Source: three-view drawing plus pictorial views. Frame: mm from the lowest corner of the part. A direction names the side the tool comes from. Coordinates: 2 decimals unless noted, no trailing zeros. Write each loop counter-clockwise with the first axis right and the second up, starting at its lowest first coordinate (ties: lowest second). Pieces come first, ordered by that corner, then holes. Notation, with made-up numbers: (19, 3.5) -> (55, 3.5) arc R22 ccw to (55, 29.5) -> close; hole circle Ø8 at (-15, 2). An arc over 180 degrees is marked (long way). One line per item, written item: value.
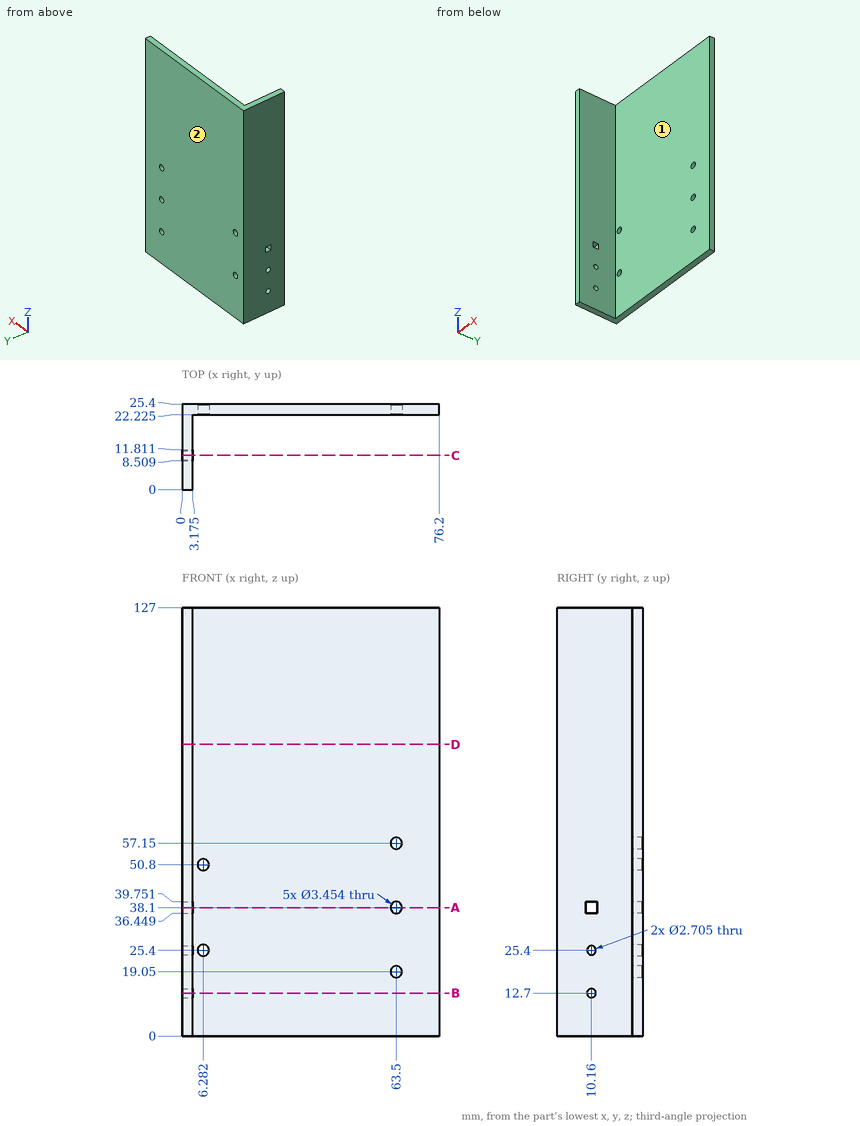
(1) Section C-C (y = 10.16). Return the cut outline in (x, z) (1 decimal).
Responses:
outline: (0, 0) -> (3.2, 0) -> (3.2, 11.3) -> (0, 11.3) -> close; (0, 14.1) -> (3.2, 14.1) -> (3.2, 24) -> (0, 24) -> close; (0, 26.8) -> (3.2, 26.8) -> (3.2, 36.4) -> (0, 36.4) -> close; (0, 39.8) -> (3.2, 39.8) -> (3.2, 127) -> (0, 127) -> close
(2) Section B-B (z = 12.7). Return the cut outline in (x, y) (1 decimal).
Responses:
outline: (0, 0) -> (3.2, 0) -> (3.2, 8.8) -> (0, 8.8) -> close; (0, 11.5) -> (3.2, 11.5) -> (3.2, 22.2) -> (76.2, 22.2) -> (76.2, 25.4) -> (0, 25.4) -> close
(3) Section D-D (z = 86.5). Return the cut outline in (x, y) (1 decimal).
Responses:
outline: (0, 0) -> (3.2, 0) -> (3.2, 22.2) -> (76.2, 22.2) -> (76.2, 25.4) -> (0, 25.4) -> close
(4) Section A-A (z = 38.1). Return the cut outline in (x, y) (1 decimal), then the cut area to 3 significant figures.
Responses:
outline: (0, 0) -> (3.2, 0) -> (3.2, 8.5) -> (0, 8.5) -> close; (0, 11.8) -> (3.2, 11.8) -> (3.2, 22.2) -> (61.8, 22.2) -> (61.8, 25.4) -> (0, 25.4) -> close; (65.2, 22.2) -> (76.2, 22.2) -> (76.2, 25.4) -> (65.2, 25.4) -> close
area: 291 mm2
(5) Reachability of the marked faces 1 and 2 from +Z, -Z, +X, -X, +Y, -Y: full face, straight path, thin tool, end or side. Return the list, or none.
Responses:
face 1: +Z, -Z, +X, -Y
face 2: +Z, -Z, +X, -X, +Y
(6) Line query: line 1 (Z direction, x = 63.5, y = 23.7); line 2 (X direction, y = 23.2, z = 19.05); line 3 (Y direction, x = 1.5, z = 12.7). Output: solid intervals per line, ascending. Write a range as [from, to].
Responses:
line 1: z = [0, 17.32], [20.78, 36.37], [39.83, 55.42], [58.88, 127]
line 2: x = [0, 61.77], [65.23, 76.2]
line 3: y = [0, 8.81], [11.51, 25.4]
(7) First-contact query: pin 1 (8 mm diameter, centred on x = 64.5, z = 54, fed in from -Y) (3 decimals); pin 2 (1 mm diameter, centred on y = 17, z = 37, fed in from -X); pin 3 (11 mm diameter, centred on y = 8.5, z = 90, fed in from +X) (3 decimals); pin 4 (3 mm diameter, centred on x = 63.5, z = 38.1, fed in from +Y). Flat tips, straight axial feed; report the tip coordinate or a pass-through.
Responses:
pin 1: stops at y = 22.225
pin 2: stops at x = 0
pin 3: stops at x = 3.175
pin 4: passes through
